For this review, take the finished solid that the model builds, in its own axes (mm). A direction names the side the tool comes from. Coordinates: 2 decimals unless noted, no trailing zeros. Write each loop counter-clockwise with the first axis right and the second up, starting at its lowest first coordinate (ties: lowest second). Pieces come first, ordered by that corner, then holes.
1) Insertion check: P1, Ø10.5, axis at x = 40, y = -11.5, coming from the +Z side; P2, Ø1.5, axis at x = -16, z = -39.5, coming from the +Y side; P3, Ø4, axis at y = -17, z = 59, coming from the +X side. Each pin has a flat end and moves straight along its axis. Give the tip position at first contact, or say it passes through.
2) Mouldability with a two-part tool opening along X and no side actions: class faces 1 (the face through (7, -21, -57.681)), 2 (the face through (84.73, -39.49, -1.91)), 3 (the face through (85.079, -17, 2)) as pulls with the +X half, pulls with the -X half, needs draft (parallel to the pull), parting line crosses it, or undercut.
3) For faces 4 (the face through (51, -30.667, 60)), 5 (the face through (-72.421, -16, 2)), 6 (the face through (-69.921, -17, 2)), list the 3-axis set-ups (+Z, -Z, +X, -X, +Y, -Y) from which the entire face can be reached by the end or side of a thin tool; tool diameter is ignored.
4) We need section A-A on x = 40. Write out the cut boundary in (y, z).
5) We need section B-B on z = 43.5. Write out the cut boundary in (x, y).
6) To check wall thickness, follow line 1 along X through (y, z) = (-16, 53); line 2 along Z through (x, y) = (28.5, -3); line 3 along Y through (x, z) = (-28, -32.5). State the ranges of each line that lie inside material, in increasing order.
7) We need section C-C on y = -10. Write out the cut boundary in (x, z).
8) We need section D-D on x = -33.5. Write out the cut boundary in (y, z).
from build123d import *

# Parameters (mm, degrees)
F0_W     = 160
F0_H     = 120
F1_DEPTH = 42.5
F2_R     = 10
F3_W     = 155
F3_H     = 110
F4_DEPTH = 35
F5_W     = 60.082482
F5_H     = 25.754019
F6_DEPTH = 5.001


with BuildPart() as f1:
    # F0 (on Front) → F1 (new body)
    with BuildSketch(Plane.XZ):
        with Locations((7.578965, 2.318726)):
            Rectangle(F0_W, F0_H)
    extrude(amount=F1_DEPTH)

    # F2
    f2_edges = [f1.edges().sort_by_distance(p)[0] for p in [
        (87.578965, -21.25, 62.318726),
        (-72.421035, -21.25, 62.318726),
        (87.578965, -21.25, -57.681274),
        (-72.421035, -21.25, -57.681274),
        (-72.421035, -42.5, 2.318726),
        (87.578965, -42.5, 2.318726),
        (7.578965, -42.5, 62.318726),
    ]]
    fillet(f2_edges, radius=F2_R)

    # F3 (on Front) → F4 (cut)
    with BuildSketch(Plane.XZ):
        with Locations((7.578965, 2.318726)):
            Rectangle(F3_W, F3_H)
    extrude(amount=F4_DEPTH, mode=Mode.SUBTRACT)

    # F5 (on face) → F6 (cut, through all)
    with BuildSketch(Plane(origin=(0, 0, 57.318726), x_dir=(1, 0, 0), z_dir=(0, 0, -1))):
        with Locations((51.495171, 17.789639)):
            Rectangle(F5_W, F5_H)
    extrude(amount=-F6_DEPTH, mode=Mode.SUBTRACT)


solid = f1.part
Result:
1. P1: stops at z = -52.68
1. P2: stops at y = -35
1. P3: stops at x = 86.42
2. face 1: needs draft
2. face 2: pulls with the +X half
2. face 3: undercut
3. face 4: +Z
3. face 5: +Z, -Z, -X, +Y, -Y
3. face 6: +Y
4. outline: (-42.5, -57.68) - (0, -57.68) - (0, -52.68) - (-35, -52.68) - (-35, 57.32) - (-30.67, 57.32) - (-30.67, 62.32) - (-32.5, 62.32) arc R10 ccw to (-42.5, 52.32) - close; (-4.91, 57.32) - (0, 57.32) - (0, 62.32) - (-4.91, 62.32) - close
5. outline: (-72.42, -32.5) arc R10 ccw to (-62.42, -42.5) - (77.58, -42.5) arc R10 ccw to (87.58, -32.5) - (87.58, 0) - (85.08, 0) - (85.08, -35) - (-69.92, -35) - (-69.92, 0) - (-72.42, 0) - close
6. line 1: x = -72.4 to -69.92, 85.08 to 87.56
6. line 2: z = -57.68 to -52.68, 57.32 to 62.32
6. line 3: y = -42.5 to -35
7. outline: (-72.42, -47.68) arc R10 ccw to (-62.42, -57.68) - (77.58, -57.68) arc R10 ccw to (87.58, -47.68) - (87.58, 52.32) arc R10 ccw to (81.54, 61.5) - (81.54, 57.32) - (85.08, 57.32) - (85.08, -52.68) - (-69.92, -52.68) - (-69.92, 57.32) - (21.45, 57.32) - (21.45, 62.32) - (-62.42, 62.32) arc R10 ccw to (-72.42, 52.32) - close
8. outline: (-42.5, -57.68) - (0, -57.68) - (0, -52.68) - (-35, -52.68) - (-35, 57.32) - (0, 57.32) - (0, 62.32) - (-32.5, 62.32) arc R10 ccw to (-42.5, 52.32) - close
